The listing builds one solid part. Answer for the finished solid, in the listing's coordinates (mm). A direction names the side the tool comes from. Give positions to 0.01 mm unless a question says otherwise; leave off trailing zeros. Write each loop counter-clockwise with the first axis right and the second up, starting at its lowest first coordinate (ties: lowest second). Pieces come first, ordered by that corner, then holes. Notation, with made-up numbers: (52, 3) - (95, 3) arc R14 ccw to (95, 18) - close; hole circle Ø7 at (84, 12). An arc over 180 degrees is marked (long way). Return JSON: item names as keys, results as strings.
from build123d import *

# Parameters (mm, degrees)
BOSS_EXTRUDE2_DEPTH             = 6.35
BOSS_EXTRUDE2_DEPTH_BACK        = 2.54
SKETCH2_W                       = 86.35999999999999
SKETCH2_H                       = 132.07999999999998
SKETCH3_W                       = 86.35999999999999
SKETCH3_H                       = 8.889999999999999
BOSS_EXTRUDE3_DEPTH             = 101.6
SKETCH6_W                       = 25.39999999999999
SKETCH6_H                       = 8.89
BOSS_EXTRUDE4_DEPTH             = 6.35
CBORE_FOR_M3_SBHCS1_D           = 3.4
CBORE_FOR_M3_SBHCS1_CBORE_D     = 6.7
CBORE_FOR_M3_SBHCS1_CBORE_DEPTH = 2.666
CUT_EXTRUDE3_DEPTH              = 182.55670546691465
CUT_EXTRUDE3_DEPTH_BACK         = 182.55670546691465
SKETCH7_R                       = 2.7940000000000107
FILLET1_R                       = 2.5399999999999996
SKETCH11_W                      = 86.35999999999999
SKETCH11_H                      = 8.889999999999999
CUT_EXTRUDE4_DEPTH              = 22.86
SKETCH12_W                      = 11.429999999999993
SKETCH12_H                      = 8.89
SKETCH12_W_2                    = 11.429999999999998
CUT_EXTRUDE5_DEPTH              = 2.5399999999999996
MOVE_START                      = 11.43
MOVE_FACE1_DEPTH                = 25.4
MOVE_START_2                    = 49.53
MOVE_FACE1_2_DEPTH              = 25.4
SKETCH13_W                      = 86.35999999999999
SKETCH13_H                      = 78.74000000000001
CUT_EXTRUDE6_DEPTH              = 190.71096594556678
CUT_EXTRUDE7_DEPTH              = 192.9171289906141
FILLET8_R                       = 2.54
BOSS_EXTRUDE6_START             = -86.36
BOSS_EXTRUDE6_DEPTH             = 86.36
BOSS_EXTRUDE8_START             = -86.36
BOSS_EXTRUDE8_DEPTH             = 86.36
CUT_EXTRUDE8_DEPTH              = 169.1443549453861
CUT_EXTRUDE8_DEPTH_BACK         = 169.1443549453861
FILLET12_R                      = 19.05
FILLET13_R                      = 25.4
FILLET14_R                      = 8.255
FILLET16_R                      = 12.7


# Read off the part's stored shape, not the designer's step: Move Face1
with BuildPart() as part:
    # Sketch2 → Boss-Extrude2 (new, two sides: drawn at the far end of the back side and taken through both)
    with BuildSketch(Plane.XY.offset(-BOSS_EXTRUDE2_DEPTH_BACK)):
        with Locations((43.17999999999999, 66.03999999999999)):
            Rectangle(SKETCH2_W, SKETCH2_H)
    extrude(amount=BOSS_EXTRUDE2_DEPTH + BOSS_EXTRUDE2_DEPTH_BACK)

    # Sketch3 → Boss-Extrude3 (add)
    with BuildSketch(Plane.XY.offset(6.35)):
        Polygon((0, 132.07999999999998), (86.35999999999999, 132.07999999999998), (86.35999999999999, 123.18999999999998), (-3.27e-15, 123.18999999999998), align=None)
        with Locations((43.17999999999999, 4.444999999999999)):
            Rectangle(SKETCH3_W, SKETCH3_H)
    extrude(amount=BOSS_EXTRUDE3_DEPTH)

    # Sketch6 → Boss-Extrude4 (add)
    with BuildSketch(Plane.XY.offset(107.94999999999999)):
        with Locations((62.23, 127.63499999999999)):
            Rectangle(SKETCH6_W, SKETCH6_H)
        with Locations((24.129999999999995, 127.63499999999999)):
            Rectangle(SKETCH6_W, SKETCH6_H)
    extrude(amount=BOSS_EXTRUDE4_DEPTH)

    # CBORE for M3 SBHCS1 (through all)
    with Locations(Plane(origin=(0, 0, -2.54), x_dir=(1, 0, 0), z_dir=(0, 0, -1))):
        with Locations((34.417, -53.721), (54.483, -53.721), (34.417, -73.787), (54.483, -73.787)):
            CounterBoreHole(CBORE_FOR_M3_SBHCS1_D / 2, CBORE_FOR_M3_SBHCS1_CBORE_D / 2, CBORE_FOR_M3_SBHCS1_CBORE_DEPTH)

    # Sketch7 → Cut-Extrude3 (cut, two sides: drawn at the far end of the back side and taken through both)
    with BuildSketch(Plane.ZY.offset(-49.53).offset(-CUT_EXTRUDE3_DEPTH_BACK)):
        with Locations((111.12499999999999, 127.635)):
            Circle(SKETCH7_R)
    extrude(amount=CUT_EXTRUDE3_DEPTH + CUT_EXTRUDE3_DEPTH_BACK, mode=Mode.SUBTRACT)

    # Fillet1
    fillet1_edges = [part.edges().sort_by_distance(p)[0] for p in [
        (62.23, 123.18999999999998, 114.29999999999998),
        (62.23, 132.07999999999998, 114.29999999999998),
        (24.129999999999995, 123.18999999999998, 114.29999999999998),
        (24.129999999999995, 132.07999999999998, 114.29999999999998),
    ]]
    fillet(fillet1_edges, radius=FILLET1_R)

    # Sketch11 → Cut-Extrude4 (cut)
    with BuildSketch(Plane.XY.offset(107.94999999999999)):
        with Locations((43.17999999999999, 4.444999999999999)):
            Rectangle(SKETCH11_W, SKETCH11_H)
    extrude(amount=-CUT_EXTRUDE4_DEPTH, mode=Mode.SUBTRACT)

    # Sketch12 → Cut-Extrude5 (cut)
    with BuildSketch(Plane.XY.offset(107.94999999999999)):
        with Locations((80.64499999999998, 127.63499999999999)):
            Rectangle(SKETCH12_W, SKETCH12_H)
        Polygon((49.53, 123.18999999999998), (36.82999999999999, 123.18999999999997), (36.82999999999999, 132.07999999999998), (49.53, 132.07999999999998), align=None)
        with Locations((5.714999999999999, 127.63499999999999)):
            Rectangle(SKETCH12_W_2, SKETCH12_H)
    extrude(amount=-CUT_EXTRUDE5_DEPTH, mode=Mode.SUBTRACT)

    # Move Face1 outline → Move Face1 (add)
    with BuildSketch(Plane.YZ.offset(MOVE_START)):
        with BuildLine():
            ThreePointArc((132.08, 113.03), (131.336051224, 114.826051224), (129.54, 115.57))
            Line((129.54, 115.57), (125.73, 115.57))
            ThreePointArc((125.73, 115.57), (123.933948776, 114.826051224), (123.19, 113.03))
            Line((123.19, 113.03), (123.19, 111.76))
            ThreePointArc((123.19, 111.76), (123.933948776, 113.556051224), (125.73, 114.3))
            Line((125.73, 114.3), (129.54, 114.3))
            ThreePointArc((129.54, 114.3), (131.336051224, 113.556051224), (132.08, 111.76))
            Line((132.08, 111.76), (132.08, 113.03))
        make_face()
    extrude(amount=MOVE_FACE1_DEPTH)

    # Move Face1 2 outline → Move Face1 2 (add)
    with BuildSketch(Plane.YZ.offset(MOVE_START_2)):
        with BuildLine():
            ThreePointArc((132.08, 113.03), (131.336051224, 114.826051224), (129.54, 115.57))
            Line((129.54, 115.57), (125.73, 115.57))
            ThreePointArc((125.73, 115.57), (123.933948776, 114.826051224), (123.19, 113.03))
            Line((123.19, 113.03), (123.19, 111.76))
            ThreePointArc((123.19, 111.76), (123.933948776, 113.556051224), (125.73, 114.3))
            Line((125.73, 114.3), (129.54, 114.3))
            ThreePointArc((129.54, 114.3), (131.336051224, 113.556051224), (132.08, 111.76))
            Line((132.08, 111.76), (132.08, 113.03))
        make_face()
    extrude(amount=MOVE_FACE1_2_DEPTH)

    # Sketch13 → Cut-Extrude6 (cut, through all)
    with BuildSketch(Plane(origin=(0, 8.889999999999999, 0), x_dir=(1, 0, 0), z_dir=(0, 1, 0))):
        with Locations((43.17999999999999, -45.72)):
            Rectangle(SKETCH13_W, SKETCH13_H)
    extrude(amount=-CUT_EXTRUDE6_DEPTH, mode=Mode.SUBTRACT)

    # Sketch14 → Cut-Extrude7 (cut, through all)
    with BuildSketch(Plane.XY.offset(6.35)):
        Polygon((86.35999999999999, 91.43999999999998), (65.40499999999999, 45.71999999999999), (20.955, 45.71999999999999), (3.89e-15, 91.43999999999998), (0, 0), (86.35999999999999, 0), align=None)
    extrude(amount=-CUT_EXTRUDE7_DEPTH, mode=Mode.SUBTRACT)

    # Fillet8
    fillet8_edges = [part.edges().sort_by_distance(p)[0] for p in [
        (80.64499999999998, 123.18999999999998, 105.40999999999998),
        (80.64499999999998, 132.07999999999998, 105.40999999999998),
        (43.17999999999999, 123.18999999999997, 105.40999999999998),
        (43.17999999999999, 132.07999999999998, 105.40999999999998),
        (5.714999999999999, 123.18999999999998, 105.40999999999998),
        (5.714999999999999, 132.07999999999998, 105.40999999999998),
    ]]
    fillet(fillet8_edges, radius=FILLET8_R)

    # Sketch17 → Boss-Extrude6 (add)
    with BuildSketch(Plane(origin=(86.35999999999999, 0, 0), x_dir=(0, 0, -1), z_dir=(1, 0, 0)).offset(BOSS_EXTRUDE6_START)):
        with BuildLine():
            Line((-102.86999999999999, 132.07999999999998), (2.5400000000000063, 132.07999999999998))
            Line((2.54, 132.07999999999998), (2.5400000000000005, 138.42999999999998))
            Line((2.539999999999999, 138.42999999999998), (-50.165, 138.42999999999998))
            ThreePointArc((-50.16499999999999, 138.43), (-76.70777431972341, 136.8342768537044), (-102.86999999999999, 132.07999999999998))
        make_face()
    extrude(amount=BOSS_EXTRUDE6_DEPTH)

    # Sketch20 → Boss-Extrude8 (add)
    with BuildSketch(Plane.ZY.offset(BOSS_EXTRUDE8_START)):
        with BuildLine():
            Line((6.35, 110.48999999999998), (6.35, 123.18999999999998))
            Line((6.35, 123.18999999999998), (102.86999999999999, 123.18999999999998))
            ThreePointArc((102.86999999999999, 123.18999999999998), (54.19402954228848, 120.00137547860714), (6.35, 110.48999999999998))
        make_face()
    extrude(amount=BOSS_EXTRUDE8_DEPTH)

    # Sketch16 → Cut-Extrude8 (cut, two sides: drawn at the far end of the back side and taken through both)
    with BuildSketch(Plane(origin=(0, 132.07999999999998, 0), x_dir=(1, 0, 0), z_dir=(0, 1, 0)).offset(-CUT_EXTRUDE8_DEPTH_BACK)):
        Polygon((10.160000000000016, -92.71), (10.160000000000016, -6.350000000000009), (76.19999999999999, -6.350000000000002), (76.19999999999999, -92.71), align=None)
    extrude(amount=CUT_EXTRUDE8_DEPTH + CUT_EXTRUDE8_DEPTH_BACK, mode=Mode.SUBTRACT)

    # Fillet12
    fillet12_edges = [part.edges().sort_by_distance(p)[0] for p in [
        (10.160000000000016, 128.681636078935, 92.71),
        (76.19999999999999, 124.45999999999998, 6.350000000000002),
        (76.19999999999999, 128.681636078935, 92.71),
        (10.160000000000016, 124.45999999999998, 6.350000000000009),
    ]]
    fillet(fillet12_edges, radius=FILLET12_R)

    # Fillet13
    fillet13_edges = [part.edges().sort_by_distance(p)[0] for p in [
        (71.755, 110.49000000000001, 6.349999999999991),
        (14.605000000000006, 110.49000000000001, 6.349999999999989),
    ]]
    fillet(fillet13_edges, radius=FILLET13_R)

    # Fillet14
    fillet14_edges = [part.edges().sort_by_distance(p)[0] for p in [
        (20.955, 45.71999999999999, 1.9049999999999994),
        (65.40499999999999, 45.71999999999999, 1.9049999999999994),
    ]]
    fillet(fillet14_edges, radius=FILLET14_R)

    # Fillet16
    # the kernel refuses this fillet: 12.7 mm, written as the material it takes off along each edge
    with BuildSketch(Plane(origin=(-31.750000000000018, 138.42999999999998, -2.5400000000000005), x_dir=(0, 0, 1), z_dir=(1, 0, 0))) as fillet16_piece_1:
        with BuildLine():
            CenterArc((FILLET16_R, FILLET16_R), FILLET16_R, 180, 90)
            Line((3.11e-15, FILLET16_R), (0, 0))
            Line((0, 0), (FILLET16_R, 0))
        make_face()
    extrude(amount=149.86, mode=Mode.SUBTRACT)


solid = part.part
Item 1: For faces 1 (the face through (6, 128, 105.41)), 2 (the face through (70.47, 129.72, 87.28)), 3 (the face through (33.69, 56.99, -1.23)), determine the directions among +Z, -Z, +X, -X, +Y, -Y from which every point of the face is accessible in a straight line to the end or side of a thin tool.
Answer below:
{"face 1": "+Z, -X, +Y, -Y", "face 2": "+Y, -Y", "face 3": "-Z"}
Item 2: A cutting plane is placed at A-A on x = 64. Determine the outline of the cut face in (y, z) (3 decimals).
Answer below:
{"outline": "(46.695, -2.54) - (125.73, -2.54) arc R12.7 ccw to (138.174, 7.624) - (98.383, 7.624) arc R25.4 cw to (90.439, 6.35) - (46.695, 6.35) - close; (123.015, 91.436) - (134.557, 91.436) arc R222.25 ccw to (132.08, 102.87) - (132.08, 113.03) arc R2.54 ccw to (129.54, 115.57) - (125.73, 115.57) arc R2.54 ccw to (123.19, 113.03) - (123.19, 102.87) arc R373.126 cw to start; hole circle Ø5.588 at (127.635, 111.125)"}
Item 3: A cutting plane is placed at C-C on x = 21. Determine the outline of the cut face in (y, z) (3 decimals).
Answer below:
{"outline": "(47.606, -2.54) - (125.73, -2.54) arc R12.7 ccw to (138.279, 8.21) - (99.98, 8.21) arc R25.4 cw to (90.439, 6.35) - (47.606, 6.35) - close; (122.996, 90.85) - (134.667, 90.85) arc R222.25 ccw to (132.08, 102.87) - (132.08, 113.03) arc R2.54 ccw to (129.54, 115.57) - (125.73, 115.57) arc R2.54 ccw to (123.19, 113.03) - (123.19, 102.87) arc R373.126 cw to start; hole circle Ø5.588 at (127.635, 111.125)"}
Item 4: A cutting plane is placed at D-D on z = 80. Determine the outline of the cut face in (x, y), then the cut area to 3 significant figures.
Answer below:
{"outline": "(0, 122.49) - (11.25, 122.49) - (11.25, 136.41) - (0, 136.41) - close; (75.11, 122.49) - (86.36, 122.49) - (86.36, 136.41) - (75.11, 136.41) - close", "area": "313 mm²"}
Item 5: The mould has two halves that part along Y. Classify faces 4 (the face through (62, 128, 115.57)), 5 (the face through (43, 45.72, 2)), 6 (the face through (36, 55, 0.126)): +Y half, -Y half, draft (parallel to the pull), parting line (faces both ways), or undercut.
Answer below:
{"face 4": "draft", "face 5": "-Y half", "face 6": "undercut"}
Item 6: Consider L1, parallel to X at y = 121.5, z = 30.5; L2, parallel to Z at x = 16.5, y = 58.5. Determine where each line is inside the solid, lowest interval first.
Answer below:
{"L1": "x = 0 to 10.16, 76.2 to 86.36", "L2": "z = -2.54 to 6.35"}
Item 7: A cutting plane is placed at B-B on z = 18. Determine the outline of the cut face in (x, y), then the cut area to 3 significant figures.
Answer below:
{"outline": "(0, 111.8) - (11.66, 111.8) - (11.66, 138.43) - (0, 138.43) - close; (74.7, 111.8) - (86.36, 111.8) - (86.36, 138.43) - (74.7, 138.43) - close", "area": "621 mm²"}
Item 8: Flat-ended cylindrical pins translate along their axes: P1, Ø1.1, axis at x = 81, y = 127, coming from the +Z side; P2, Ø4.5, axis at x = 34.417, y = 53.721, coming from the -Z side; P3, Ø2, axis at x = 75.5, y = 103.5, coming from the +Z side. Find the tip coordinate at first contact, or state that the pin passes through.
Answer below:
{"P1": "stops at z = 105.41", "P2": "stops at z = 0.13", "P3": "stops at z = 10.6"}
